Autodesk Inventor part; units mm, degrees
sketch "Sketch2" plane through (0, 0, 0) normal (0, 1, 0) x (-1, 0, 0)
  line L0 (0, -87.5) -> (-250, -87.5)
  line L1 (-250, -87.5) -> (-250, 87.5)
  line L2 (-250, 87.5) -> (0, 87.5)
  line L3 (0, 87.5) -> (0, -87.5)
  line L4 (0, -122.5) -> (0, 122.5)
  line L5 (-300, 0) -> (50, 0)
  point P0 (0, 0)
  dimension "d0" = 0
  dimension "d1" = 250
  dimension "d2" = 175
  dimension "d3" = 87.5
extrude "Extrusion1" add sketch "Sketch2" along normal blind 120
chamfer "Chamfer1" distance 175 angle 30 1 edges at (250, 60, 87.5) measured on face at (83.3333, 40, 87.5)
chamfer "Chamfer2" distance 160 angle 30 1 edges at (250, 120, -50.5181) measured on face at (108.3333, 120, -4.5121)
sketch "Sketch4" plane through (0, 0, 87.5) normal (0, 0, 1) x (1, 0, 0)
  line L0 (0, 65) -> (20, 65)
  line L1 (20, 65) -> (20, 35)
  line L2 (20, 35) -> (0, 35)
  line L3 (0, 35) -> (0, 65)
  line L4 (0, 144) -> (0, -24)
  line L5 (-50, 0) -> (300, 0)
  point P0 (0, 0)
  dimension "d15" = 0
  dimension "d16" = 30
  dimension "d17" = 20
  dimension "d18" = 35
sketch "Sketch6" plane through (0, 0, 87.5) normal (0, 0, 1) x (1, 0, 0)
  circle A0 centre (50, 25) radius 10
  line L0 (-50, 0) -> (300, 0)
  line L1 (0, 144) -> (0, -24)
  point P0 (0, 0)
  dimension "d23" = 20
  dimension "d24" = 25
  dimension "d25" = 50
sketch "Sketch7" plane through (250, 0, -87.5) normal (0, 0, -1) x (-1, 0, 0)
  line L0 (230, 35) -> (250, 35)
  line L1 (250, 65) -> (230, 65)
  line L2 (230, 65) -> (230, 35)
  point P0 (250, 0)
extrude "Extrusion3" cut sketch "Sketch4" against normal up to next
extrude "Extrusion4" cut sketch "Sketch6" against normal up to surface (175 mm away)
sketch "Sketch8" plane through (0, 120, 0) normal (0, 1, 0) x (1, 0, 0)
  circle A0 centre (40, 62.5) radius 10
  line L0 (90, 87.5) -> (0, 87.5)
  line L1 (0, 87.5) -> (0, -87.5)
  point P0 (0, 0)
  dimension "d28" = 20
  dimension "d29" = 25
  dimension "d30" = 40
extrude "Extrusion5" cut sketch "Sketch8" against normal up to surface (120 mm away)
sketch "Sketch9" plane through (0, 120, 0) normal (0, 1, 0) x (1, 0, 0)
  line L0 (0, 37.5) -> (250, 37.5)
  line L1 (250, 37.5) -> (250, -37.5)
  line L2 (250, -37.5) -> (0, -37.5)
  line L3 (0, -37.5) -> (0, 37.5)
  line L4 (90, 87.5) -> (0, 87.5)
  line L5 (0, 87.5) -> (0, -87.5)
  point P0 (0, 0)
  dimension "d33" = 50
  dimension "d34" = 75
  dimension "d35" = 0
  dimension "d36" = 250
extrude "Extrusion6" cut sketch "Sketch9" against normal blind 25
equation "\"d3\" = 0.5 * d2"
properties part number "chap3ex3"
Part model, mm, in its own coordinate system. A direction names the side the tool comes from. Round coordinates to 2 decimals unless told otherwise and drop trailing zeros. Write each loop counter-clockwise with the first axis right and the second up, starting at its lowest first coordinate (ties: lowest second). Pieces come first, ordered by that corner, then holes.
Item 1: Two-plate mould, pull along Y, no slides. Class faces 1 (the flat face through (10, 35, 1)), 2 (the flat face through (250, 14, -51)), 3 (the flat face through (56, 120, -62)): +Y half, -Y half, draft (parallel to the pull), parting line (faces both ways), or undercut.
Results:
face 1: undercut
face 2: draft
face 3: +Y half
Item 2: Which spindle directions (+Z, -Z, +X, -X, +Y, -Y) get a long thin tool onto all of the face, cutting with end or side? Do faces 4 (the flat face through (66, 95, -1)), 5 (the flat face through (20, 50, 1)), 6 (the flat face through (0, 17, 1)). Say none if no direction does.
Results:
face 4: +X, -X, +Y
face 5: +Z, -Z, -X
face 6: +Z, -Z, -X, +Y, -Y
Item 3: Cut at A-A, the plane z = -62.5. Give the cut face in (x, y).
Results:
outline: (0, 0) - (30, 0) - (30, 120) - (0, 120) - (0, 65) - (20, 65) - (20, 35) - (0, 35) - close; (50, 0) - (250, 0) - (250, 27.62) - (90, 120) - (50, 120) - (50, 35) arc R10 cw to (50, 15) - close
Item 4: Probe L1, parallel to Z at x = 40, y = 51; L2, parallel to Y at x = 50, z = 41.5; L3, parallel to Y at x = 50, z = -29. List the from-to ranges inside material, lowest first.
Results:
L1: z = -87.5 to -72.5, -52.5 to 87.5
L2: y = 0 to 15, 35 to 120
L3: y = 0 to 15, 35 to 95
Item 5: Cut at C-C, the plane y = 25. Give the cut face in (x, z).
Results:
outline: (0, -87.5) - (40, -87.5) - (40, -72.5) arc R10 cw to (40, -52.5) - (40, 87.5) - (0, 87.5) - close; (60, -87.5) - (250, -87.5) - (250, -13.54) - (75, 87.5) - (60, 87.5) - close
Item 6: Cut at D-D, the plane z = 47. Give the cut face in (x, y), plus the area to 3 significant figures.
Results:
outline: (0, 0) - (145.15, 0) - (145.15, 88.16) - (90, 120) - (0, 120) - (0, 65) - (20, 65) - (20, 35) - (0, 35) - close; hole circle Ø20 at (50, 25)
area: 15,600 mm2
Item 7: Cut at B-B, the plane x = 36.5. Give the cut face in (y, z).
Results:
outline: (0, -87.5) - (120, -87.5) - (120, -71.87) - (0, -71.87) - close; (0, -53.13) - (120, -53.13) - (120, -37.5) - (95, -37.5) - (95, 37.5) - (120, 37.5) - (120, 87.5) - (0, 87.5) - close
Item 8: Drop flat-ended pins along their axis: pin 1 Ø10 at (x, z) = (9.5, 32) entering from +Y; pin 2 Ø2 at (x, z) = (96, 46) entering from +Y; pin 3 Ø3 at (y, z) = (85, -44.5) entering from +X. Give the stop position or say it passes through.
Results:
pin 1: stops at y = 95
pin 2: stops at y = 117.11
pin 3: stops at x = 153.22
